Print and shaded views of the part. All mm, measured from the part's lowest x, y and z. A direction names the side the tool comes from. Coordinates: 2 decimals unless noted, no trailing zeros. Loops run counter-clockwise (first coordinate to the right, second up) from the corner with the lowest first, then second, coordinate; pieces in that order, holes last. Notation, with made-up numbers: M 42.5,69 L 101.5,69 A3 ccw 101.5,74 Z; hole C 7.5,49 d9. An arc over 180 degrees is marked long. Use a Markdown table: item, result. Add a question column.
1) Band-saw the part on D-D (y = 3). List the corners of the cut face in (x, z), plus the area to 3 significant figures.
2) Band-saw the part on A-A (z = 37.5). List the corners of the cut face in (x, y), plus the area to 3 significant figures.
3) Wall check: probe 1 along X at (y, z) = (30, 37.5); probe 2 along X at (y, z) = (8, 37.5); probe 3 along Y at (x, z) = (25.5, 19.5). Give the ranges that are in metal, low to high. Write a range as from..to.
4) Band-saw the part on C-C (y = 29). List the corners of the cut face in (x, z).
5) Band-saw the part on B-B (x = 37.5). List the corners of the cut face in (y, z), plus the area to 3 significant figures.
6) Pin check, flat tips, straight feed: pin 1 Ø5 at (x, y) = (42.5, 23) entering from +Z; pin 2 Ø3 at (x, z) = (61.5, 32.5) entering from +Y; pin 3 Ø10 at (x, y) = (15.5, 28.5) entering from -Z; pin 4 Ø4 at (x, y) = (19, 28) entering from -Z. Stop position of each tip, or through.
7) Tool access for the marked faces 1 and 2: list every direction of +Z, -Z, +X, -X, +Y, -Y with a clear straight run to the whole face (end or side of a thin tool).
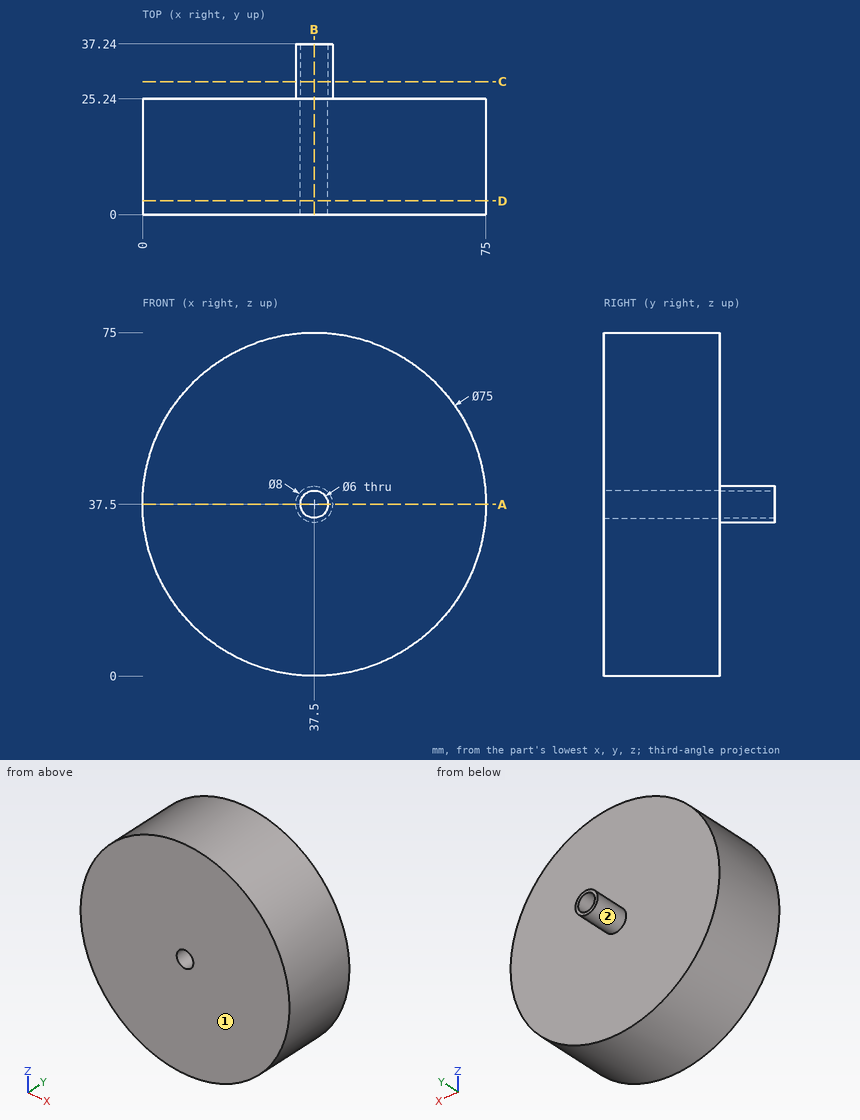
Entries:
| question | item | result |
|---|---|---|
| 1 | outline | C 37.5,37.5 d75; hole C 37.5,37.5 d6 |
| 1 | area | 4,390 mm2 |
| 2 | outline | M 0,0 L 34.5,0 L 34.5,37.24 L 33.5,37.24 L 33.5,25.24 L 0,25.24 Z; M 40.5,0 L 75,0 L 75,25.24 L 41.5,25.24 L 41.5,37.24 L 40.5,37.24 Z |
| 2 | area | 1,770 mm2 |
| 3 | probe 1 | 33.5..34.5, 40.5..41.5 |
| 3 | probe 2 | 0..34.5, 40.5..75 |
| 3 | probe 3 | 0..25.24 |
| 4 | outline | C 37.5,37.5 d8; hole C 37.5,37.5 d6 |
| 5 | outline | M 0,0 L 25.24,0 L 25.24,33.5 L 37.24,33.5 L 37.24,34.5 L 0,34.5 Z; M 0,40.5 L 37.24,40.5 L 37.24,41.5 L 25.24,41.5 L 25.24,75 L 0,75 Z |
| 5 | area | 1,770 mm2 |
| 6 | pin 1 | z = 74.92 |
| 6 | pin 2 | y = 25.24 |
| 6 | pin 3 | z = 4.72 |
| 6 | pin 4 | through |
| 7 | face 1 | +Z, -Z, +X, -X, -Y |
| 7 | face 2 | +Y |
